```python
from build123d import *

# Parameters (mm, degrees)
SKETCH2_R           = 25
BOSS_EXTRUDE1_DEPTH = 4
SKETCH3_W           = 10
SKETCH3_H           = 17
BOSS_EXTRUDE2_DEPTH = 6
FILLET1_START       = -8.5
FILLET1_DEPTH       = 17
FILLET1_START_2     = -10.744562747
FILLET1_2_DEPTH     = 21.489125494
FILLET1_START_3     = -15
FILLET1_3_DEPTH     = 30
SKETCH4_R           = 1.55
CUT_EXTRUDE1_DEPTH  = 37.742346142
SKETCH5_R           = 2.9
CUT_EXTRUDE2_DEPTH  = 6.1
FILLET2_R           = 1


with BuildPart() as part:
    # Sketch2 → Boss-Extrude1 (new body)
    with BuildSketch(Plane(origin=(0, 0, 0), x_dir=(1, 0, 0), z_dir=(0, 1, 0))):
        with Locations(Location((0, 0, 0), (0, 0, 270))):
            Circle(SKETCH2_R)
    extrude(amount=BOSS_EXTRUDE1_DEPTH)

    # Sketch3 → Boss-Extrude2 (add)
    with BuildSketch(Plane(origin=(0, 4, 0), x_dir=(1, 0, 0), z_dir=(0, 1, 0))):
        Rectangle(SKETCH3_W, SKETCH3_H)
    extrude(amount=BOSS_EXTRUDE2_DEPTH)

    # Fillet1: read off the stored shape, not the designer's step
    # Fillet1 outline → Fillet1 (add)
    with BuildSketch(Plane.XY.offset(FILLET1_START)):
        with BuildLine():
            Line((-10.744562647, 4), (-5, 4))
            Line((-5, 4), (-5, 10))
            add(Edge.make_bspline(
                [(-5, 10), (-9.177863743, 4), (-10.744562647, 4)],
                knots=[0, 0, 0, 1, 1, 1], degree=2, weights=[1, 0.88640526, 1]))
        make_face()
        with BuildLine():
            add(Edge.make_bspline(
                [(5, 10), (9.177863743, 4), (10.744562647, 4)],
                knots=[0, 0, 0, 1, 1, 1], degree=2, weights=[1, 0.88640526, 1]))
            Line((5, 10), (5, 4))
            Line((5, 4), (10.744562647, 4))
        make_face()
    extrude(amount=FILLET1_DEPTH)

    # Fillet1 2 outline → Fillet1 2 (add)
    with BuildSketch(Plane.YZ.offset(FILLET1_START_2)):
        with BuildLine():
            Line((4, 14.244562647), (4, 8.5))
            Line((4, 8.5), (10, 8.5))
            add(Edge.make_bspline(
                [(10, 8.5), (4, 12.677863743), (4, 14.244562647)],
                knots=[0, 0, 0, 1, 1, 1], degree=2, weights=[1, 0.88640526, 1]))
        make_face()
        with BuildLine():
            add(Edge.make_bspline(
                [(10, -8.5), (4, -12.677863743), (4, -14.244562647)],
                knots=[0, 0, 0, 1, 1, 1], degree=2, weights=[1, 0.88640526, 1]))
            Line((10, -8.5), (4, -8.5))
            Line((4, -8.5), (4, -14.244562647))
        make_face()
    extrude(amount=FILLET1_2_DEPTH)

    # Fillet1 3 outline → Fillet1 3 (cut)
    with BuildSketch(Plane.XY.offset(FILLET1_START_3)):
        with BuildLine():
            add(Edge.make_bspline(
                [(5, 10), (9.177863743, 4), (10.744562647, 4)],
                knots=[0, 0, 0, 1, 1, 1], degree=2, weights=[1, 0.88640526, 1]))
            Line((10.744562647, 4), (10.744562747, 10))
            Line((10.744562747, 10), (5, 10))
        make_face()
        with BuildLine():
            add(Edge.make_bspline(
                [(-5, 10), (-9.177863743, 4), (-10.744562647, 4)],
                knots=[0, 0, 0, 1, 1, 1], degree=2, weights=[1, 0.88640526, 1]))
            Line((-5, 10), (-10.744562747, 10))
            Line((-10.744562747, 10), (-10.744562647, 4))
        make_face()
    extrude(amount=FILLET1_3_DEPTH, mode=Mode.SUBTRACT)

    # Sketch4 → Cut-Extrude1 (cut, through all)
    with BuildSketch(Plane(origin=(0, 10, 0), x_dir=(1, 0, 0), z_dir=(0, 1, 0))):
        with Locations(Location((0, 3.5, 0), (0, 0, 270))):
            Circle(SKETCH4_R)
        with Locations(Location((0, -3.5, 0), (0, 0, 90))):
            Circle(SKETCH4_R)
    extrude(amount=-CUT_EXTRUDE1_DEPTH, mode=Mode.SUBTRACT)

    # Sketch5 → Cut-Extrude2 (cut)
    with BuildSketch(Plane.XZ):
        with Locations(Location((0, 3.5, 0), (0, 0, 270))):
            Circle(SKETCH5_R)
        with Locations(Location((0, -3.5, 0), (0, 0, 90))):
            Circle(SKETCH5_R)
    extrude(amount=-CUT_EXTRUDE2_DEPTH, mode=Mode.SUBTRACT)

    # Fillet2
    fillet2_edges = [part.edges().sort_by_distance(p)[0] for p in [
        (0, 0, -25),
        (0, 4, -25),
    ]]
    fillet(fillet2_edges, radius=FILLET2_R)


solid = part.part
```
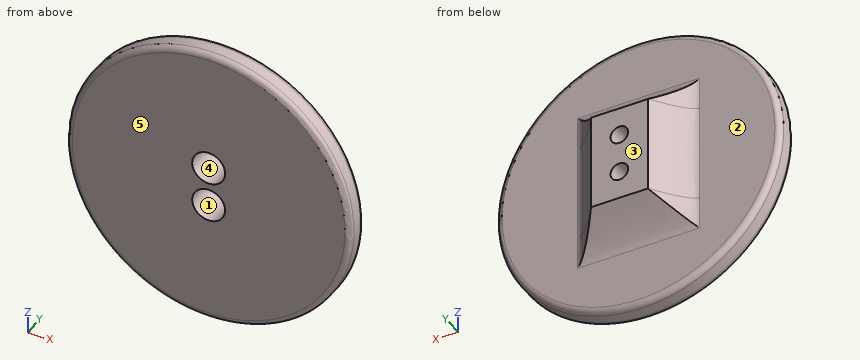
Could you check a few things on this model? Use its own coordinates, in mm. Face numbers are marked on the shaded views. A direction names the side the tool comes from. Round coordinates to 2 decimals unless told otherwise and drop trailing zeros. Write each question's results on one line, items separated by ' | '. Start each with the question number.
1. I need wall thicknesses on L1, parallel to Y at x = -2, z = -15; L2, parallel to X at y = 3.75, z = 3.5; L3, parallel to X at y = 2.5, z = 0. Which ranges of each line are inside material? Lowest first, please. Write a range as from..to.
2. I'm going to push flat-ended pins straight in: pin 1 Ø1.5 at (y, z) = (8.5, 5.5) entering from -X; pin 2 Ø6 at (y, z) = (5, 6) entering from +X; pin 3 Ø2 at (x, z) = (8, 18.5) entering from +Y; pin 4 Ø2.5 at (x, z) = (0, -3.5) entering from -Y. Where does each tip first touch, or does it pass through?
3. Imagine slicing it at A-A on x = 0. Count the separate pieces of the cut face and the enclosed holes in it, and give its area (3 significant figures).
4. Thinking about a two-plate mould opening in Z: for the marked faces 4 and 5, which applies, +Z half, -Z half, draft (parallel to the pull), parting line (faces both ways), or undercut?
5. On a 3-axis mill with a long thin cutter (end or side, diameter ignored), from which of +Z, -Z, +X, -X, +Y, -Y can I reach the whole of each face in a straight line? I mean the marked faces 1, 2 and 3. Say none if no direction works.
Result sheet:
1) L1: y = 0..4 | L2: x = -24.41..-2.9, 2.9..24.41 | L3: x = -25..25
2) pin 1: stops at x = -6.65 | pin 2: stops at x = 24.72 | pin 3: stops at y = 4 | pin 4: passes through
3) separate pieces: 3 | enclosed holes: 0 | area: 235 mm^2
4) face 4: undercut | face 5: draft
5) face 1: -Y | face 2: +Y | face 3: +Z, -Z, +X, -X, +Y
